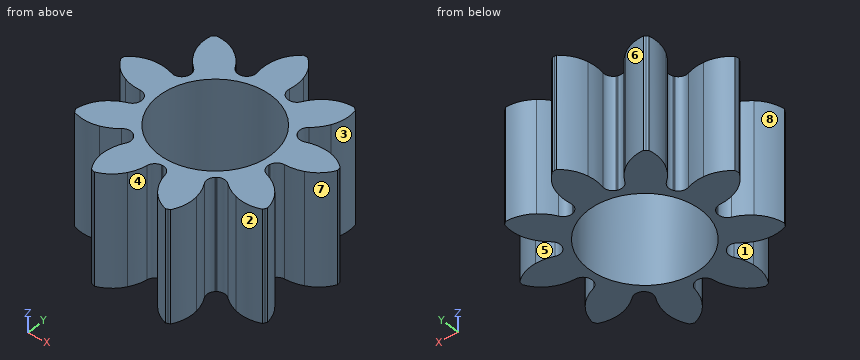
from build123d import *

# Parameters (mm, degrees)
F0_R     = 5
F1_DEPTH = 10


with BuildPart() as f1:
    # F0 (on Top) → F1 (new body)
    with BuildSketch(Plane.XY):
        with BuildLine():
            ThreePointArc((1.864316, 5.3522), (1.490455, 5.713083), (1.417156, 6.227511))
            ThreePointArc((1.417156, 6.227511), (1.483836, 7.003606), (1.389552, 7.776834))
            ThreePointArc((1.389552, 7.776834), (0.955753, 8.832789), (0.188574, 9.678163))
            Line((0.188574, 9.678163), (0, 9.68))
            Line((0, 9.68), (-0.188574, 9.678163))
            ThreePointArc((-0.188574, 9.678163), (-0.955753, 8.832789), (-1.389552, 7.776834))
            ThreePointArc((-1.389552, 7.776834), (-1.483836, 7.003606), (-1.417156, 6.227511))
            ThreePointArc((-1.417156, 6.227511), (-1.490455, 5.713083), (-1.864316, 5.3522))
            ThreePointArc((-1.864316, 5.3522), (-1.900395, 5.336418), (-1.937206, 5.32243))
            ThreePointArc((-1.937206, 5.32243), (-1.974396, 5.309483), (-2.012179, 5.298382))
            ThreePointArc((-2.012179, 5.298382), (-2.530544, 5.334521), (-2.917363, 5.68148))
            ThreePointArc((-2.917363, 5.68148), (-3.365147, 6.318865), (-3.934394, 6.850587))
            ThreePointArc((-3.934394, 6.850587), (-4.945458, 7.380655), (-6.076547, 7.535116))
            Line((-6.076547, 7.535116), (-6.222184, 7.41531))
            Line((-6.222184, 7.41531), (-6.365459, 7.29269))
            ThreePointArc((-6.365459, 7.29269), (-6.409757, 6.151962), (-6.063311, 5.064213))
            ThreePointArc((-6.063311, 5.064213), (-5.638516, 4.411282), (-5.088571, 3.85962))
            ThreePointArc((-5.088571, 3.85962), (-4.814053, 3.418429), (-4.868477, 2.901664))
            ThreePointArc((-4.868477, 2.901664), (-4.88597, 2.866383), (-4.905178, 2.832006))
            ThreePointArc((-4.905178, 2.832006), (-4.925345, 2.798183), (-4.947153, 2.765393))
            ThreePointArc((-4.947153, 2.765393), (-5.367473, 2.459878), (-5.886814, 2.477022))
            ThreePointArc((-5.886814, 2.477022), (-6.63954, 2.677457), (-7.417393, 2.718875))
            ThreePointArc((-7.417393, 2.718875), (-8.532634, 2.475031), (-9.498384, 1.866304))
            Line((-9.498384, 1.866304), (-9.532939, 1.680914))
            Line((-9.532939, 1.680914), (-9.563876, 1.494886))
            ThreePointArc((-9.563876, 1.494886), (-8.864564, 0.592564), (-7.899979, -0.018009))
            ThreePointArc((-7.899979, -0.018009), (-7.154871, -0.24513), (-6.378987, -0.31423))
            ThreePointArc((-6.378987, -0.31423), (-5.885103, -0.475745), (-5.594623, -0.906593))
            ThreePointArc((-5.594623, -0.906593), (-5.585346, -0.944864), (-5.577963, -0.983545))
            ThreePointArc((-5.577963, -0.983545), (-5.571671, -1.022419), (-5.567299, -1.061555))
            ThreePointArc((-5.567299, -1.061555), (-5.692902, -1.56577), (-6.10176, -1.886463))
            ThreePointArc((-6.10176, -1.886463), (-6.807219, -2.216763), (-7.429712, -2.685029))
            ThreePointArc((-7.429712, -2.685029), (-8.127296, -3.588688), (-8.475822, -4.675772))
            Line((-8.475822, -4.675772), (-8.383126, -4.84))
            Line((-8.383126, -4.84), (-8.287248, -5.002391))
            ThreePointArc((-8.287248, -5.002391), (-7.171543, -5.244101), (-6.04016, -5.091804))
            ThreePointArc((-6.04016, -5.091804), (-5.323383, -4.786843), (-4.684605, -4.341048))
            ThreePointArc((-4.684605, -4.341048), (-4.202447, -4.147313), (-3.702983, -4.290645))
            ThreePointArc((-3.702983, -4.290645), (-3.671276, -4.313999), (-3.640757, -4.338885))
            ThreePointArc((-3.640757, -4.338885), (-3.610949, -4.364619), (-3.582444, -4.391789))
            ThreePointArc((-3.582444, -4.391789), (-3.354559, -4.858776), (-3.461625, -5.36725))
            ThreePointArc((-3.461625, -5.36725), (-3.789724, -6.073735), (-3.965586, -6.832579))
            ThreePointArc((-3.965586, -6.832579), (-3.919106, -7.973219), (-3.487328, -9.030002))
            Line((-3.487328, -9.030002), (-3.310755, -9.096225))
            Line((-3.310755, -9.096225), (-3.132925, -9.158994))
            ThreePointArc((-3.132925, -9.158994), (-2.122877, -8.626993), (-1.354082, -7.783088))
            ThreePointArc((-1.354082, -7.783088), (-1.001025, -7.088739), (-0.798243, -6.336642))
            ThreePointArc((-0.798243, -6.336642), (-0.55342, -5.878307), (-0.078676, -5.667056))
            ThreePointArc((-0.078676, -5.667056), (-0.039376, -5.664566), (0, -5.664012))
            ThreePointArc((0, -5.664012), (0.039376, -5.664566), (0.078676, -5.667056))
            ThreePointArc((0.078676, -5.667056), (0.55342, -5.878307), (0.798243, -6.336642))
            ThreePointArc((0.798243, -6.336642), (1.001025, -7.088739), (1.354082, -7.783088))
            ThreePointArc((1.354082, -7.783088), (2.122877, -8.626993), (3.132925, -9.158994))
            Line((3.132925, -9.158994), (3.310755, -9.096225))
            Line((3.310755, -9.096225), (3.487328, -9.030002))
            ThreePointArc((3.487328, -9.030002), (3.919106, -7.973219), (3.965586, -6.832579))
            ThreePointArc((3.965586, -6.832579), (3.789724, -6.073735), (3.461625, -5.36725))
            ThreePointArc((3.461625, -5.36725), (3.354559, -4.858776), (3.582444, -4.391789))
            ThreePointArc((3.582444, -4.391789), (3.610949, -4.364619), (3.640757, -4.338885))
            ThreePointArc((3.640757, -4.338885), (3.671276, -4.313999), (3.702983, -4.290645))
            ThreePointArc((3.702983, -4.290645), (4.202447, -4.147313), (4.684605, -4.341048))
            ThreePointArc((4.684605, -4.341048), (5.323383, -4.786843), (6.04016, -5.091804))
            ThreePointArc((6.04016, -5.091804), (7.171543, -5.244101), (8.287248, -5.002391))
            Line((8.287248, -5.002391), (8.383126, -4.84))
            Line((8.383126, -4.84), (8.475822, -4.675772))
            ThreePointArc((8.475822, -4.675772), (8.127296, -3.588688), (7.429712, -2.685029))
            ThreePointArc((7.429712, -2.685029), (6.807219, -2.216763), (6.10176, -1.886463))
            ThreePointArc((6.10176, -1.886463), (5.692902, -1.56577), (5.567299, -1.061555))
            ThreePointArc((5.567299, -1.061555), (5.571671, -1.022419), (5.577963, -0.983545))
            ThreePointArc((5.577963, -0.983545), (5.585346, -0.944864), (5.594623, -0.906593))
            ThreePointArc((5.594623, -0.906593), (5.885103, -0.475745), (6.378987, -0.31423))
            ThreePointArc((6.378987, -0.31423), (7.154871, -0.24513), (7.899979, -0.018009))
            ThreePointArc((7.899979, -0.018009), (8.864564, 0.592564), (9.563876, 1.494886))
            Line((9.563876, 1.494886), (9.532939, 1.680914))
            Line((9.532939, 1.680914), (9.498384, 1.866304))
            ThreePointArc((9.498384, 1.866304), (8.532634, 2.475031), (7.417393, 2.718875))
            ThreePointArc((7.417393, 2.718875), (6.63954, 2.677457), (5.886814, 2.477022))
            ThreePointArc((5.886814, 2.477022), (5.367473, 2.459878), (4.947153, 2.765393))
            ThreePointArc((4.947153, 2.765393), (4.925345, 2.798183), (4.905178, 2.832006))
            ThreePointArc((4.905178, 2.832006), (4.88597, 2.866383), (4.868477, 2.901664))
            ThreePointArc((4.868477, 2.901664), (4.814053, 3.418429), (5.088571, 3.85962))
            ThreePointArc((5.088571, 3.85962), (5.638516, 4.411282), (6.063311, 5.064213))
            ThreePointArc((6.063311, 5.064213), (6.409757, 6.151962), (6.365459, 7.29269))
            Line((6.365459, 7.29269), (6.222184, 7.41531))
            Line((6.222184, 7.41531), (6.076547, 7.535116))
            ThreePointArc((6.076547, 7.535116), (4.945458, 7.380655), (3.934394, 6.850587))
            ThreePointArc((3.934394, 6.850587), (3.365147, 6.318865), (2.917363, 5.68148))
            ThreePointArc((2.917363, 5.68148), (2.530544, 5.334521), (2.012179, 5.298382))
            ThreePointArc((2.012179, 5.298382), (1.974396, 5.309483), (1.937206, 5.32243))
            ThreePointArc((1.937206, 5.32243), (1.900395, 5.336418), (1.864316, 5.3522))
        make_face()
        Circle(F0_R, mode=Mode.SUBTRACT)
    extrude(amount=F1_DEPTH)


solid = f1.part
Can you work these out from the model? Positions are in its coordinate system, mm. Face numbers are marked on the shaded views. A direction names the side the tool comes from. Coordinates: 2 decimals unless noted, no trailing zeros. Order: outer loops, then holes, each group sorted by start corner. A loop starts at its lowest first (then second) coordinate and runs counter-clockwise, first axis right, second up. Notation, with made-up numbers: M -26.75,47.5 L 21.25,47.5 A36 cw 21.25,85.5 Z; hole C 33,18 d9. An arc over 180 degrees is marked long. Write item = value, one per line.
(1) For pin 1 Ø1 at (x, z) = (-7, 5) entering from -Y; pin 2 Ø3 at (x, z) = (3.5, 5) entering from +Y; pin 3 Ø1 at (x, y) = (2.5, -2.5) entering from -Z; pin 4 Ø1 at (y, z) = (-5, 4) entering from +X, each with a flat end and sliding along its axis, tell me the tip position at first contact or that it passes through.
Results are:
pin_1 = -5.25
pin_2 = 7.4
pin_3 = through
pin_4 = 8.48
(2) If we mould it in two halves opening along X, with no side actions, what happens to the marked faces 1, 2 and 3? For each: pulls with the +X half, pulls with the -X half, needs draft (parallel to the pull), parting line crosses it, or undercut.
Results are:
face_1 = pulls with the -X half
face_2 = undercut
face_3 = pulls with the +X half
(3) I need wall thicknesses on line 1 along X through (y, z) = (7, 3.75); line 2 along X through (y, z) = (-4.5, 4.25); line 3 along X through (y, z) = (6, 7.75). Which ranges of each line are inside material? Lowest first, please. Write a range as [from, to].
Results are:
line_1 = [-6.41, -4.14], [-1.48, 1.48], [4.14, 6.41]
line_2 = [-8.45, -4.88], [-3.49, -2.18], [2.18, 3.49], [4.88, 8.45]
line_3 = [-6.39, -3.12], [-1.41, 1.41], [3.12, 6.39]
(4) Suppose I cut it at A-A on y = 0.25. Please give me the cut outline in (x, z), plus the area to 3 significant figures.
Results are:
outline = M -8.42,0 L -4.99,0 L -4.99,10 L -8.42,10 Z; M 4.99,0 L 8.42,0 L 8.42,10 L 4.99,10 Z
area = 68.4 mm2
(5) For the marked faces 4, 5, 6, 7 and 8, which set-ups out of +Z, -Z, +X, -X, +Y, -Y let a thin tool reach every point of the face, with its end or its side?
Results are:
face_4 = +Z, -Z, -Y
face_5 = +Z, -Z
face_6 = +Z, -Z, +Y
face_7 = +Z, -Z, +X
face_8 = +Z, -Z, -X
